Design review of the part built by this model. Coordinates are the model's own, in mm. Face numbers are marked on the shaded views. A direction names the side the tool comes from. Coordinates: 2 decimals unless noted, no trailing zeros. Write each loop counter-clockwise with the first axis right and the second up, starting at its lowest first coordinate (ties: lowest second). Pieces come first, ordered by that corner, then holes. Notation, with made-up numbers: M 59.25,52.5 L 100.25,52.5 A5 ccw 100.25,59.5 Z; hole C -19.75,39.25 d6. An arc over 180 degrees is marked long. Write item = value, one per line.
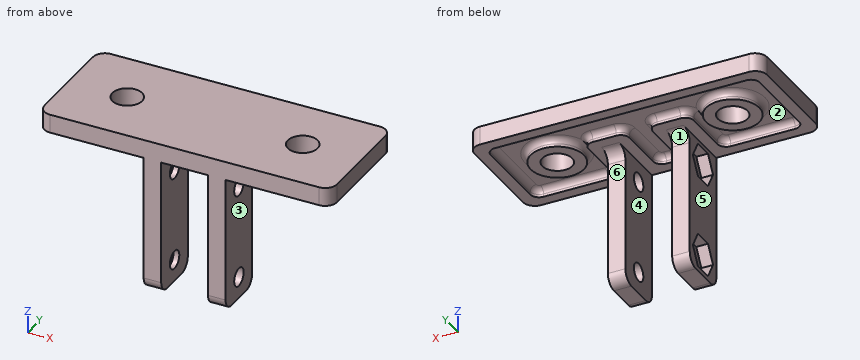
```python
from build123d import *

# Parameters (mm, degrees)
SKETCH1_W           = 50
SKETCH1_H           = 20
SKETCH1_R           = 2.55
BOSS_EXTRUDE1_DEPTH = 3.175
BOSS_EXTRUDE2_START = 4
SKETCH3_W           = 26.5
SKETCH3_H           = 8.75
SKETCH3_R           = 1.55
BOSS_EXTRUDE2_DEPTH = 3
CUT_EXTRUDE1_START  = -7
SKETCH3_3_R         = 1.55
CUT_EXTRUDE1_DEPTH  = 2
FILLET1_R           = 2
FILLET2_R           = 2
SKETCH4_R           = 4.55
CUT_EXTRUDE2_DEPTH  = 1.5
FILLET3_R           = 1.5
FILLET4_R           = 1


with BuildPart() as part:
    # Sketch1 → Boss-Extrude1 (new body)
    with BuildSketch(Plane.XY):
        Rectangle(SKETCH1_W, SKETCH1_H)
        with Locations((-15, 0)):
            Circle(SKETCH1_R, mode=Mode.SUBTRACT)
        with Locations((15, 0)):
            Circle(SKETCH1_R, mode=Mode.SUBTRACT)
    extrude(amount=BOSS_EXTRUDE1_DEPTH)

    # Sketch3 → Boss-Extrude2 (add)
    # profile 1 of 3: a face of its own
    with BuildSketch(Plane(origin=(0, 0, 0), x_dir=(0, 0, -1), z_dir=(1, 0, 0)).offset(BOSS_EXTRUDE2_START)):
        with Locations((10.075, -5.625)):
            Rectangle(SKETCH3_W, SKETCH3_H)
        Polygon((22.475, -7.259882024), (22.475, -3.940117976), (19.6, -2.280235952), (16.725, -3.940117976), (16.725, -7.259882024), (19.6, -8.919764048), align=None, mode=Mode.SUBTRACT)
        Polygon((6.475, -7.259882024), (6.475, -3.940117976), (3.6, -2.280235952), (0.725, -3.940117976), (0.725, -7.259882024), (3.6, -8.919764048), align=None, mode=Mode.SUBTRACT)
    # profile 2 of 3: a face of its own
    with BuildSketch(Plane(origin=(0, 0, 0), x_dir=(0, 0, -1), z_dir=(1, 0, 0)).offset(BOSS_EXTRUDE2_START)):
        Polygon((3.6, -8.919764048), (6.475, -7.259882024), (6.475, -3.940117976), (3.6, -2.280235952), (0.725, -3.940117976), (0.725, -7.259882024), align=None)
        with Locations((3.6, -5.6)):
            Circle(SKETCH3_R, mode=Mode.SUBTRACT)
    # profile 3 of 3: a face of its own
    with BuildSketch(Plane(origin=(0, 0, 0), x_dir=(0, 0, -1), z_dir=(1, 0, 0)).offset(BOSS_EXTRUDE2_START)):
        Polygon((19.6, -8.919764048), (22.475, -7.259882024), (22.475, -3.940117976), (19.6, -2.280235952), (16.725, -3.940117976), (16.725, -7.259882024), align=None)
        with Locations((19.6, -5.6)):
            Circle(SKETCH3_R, mode=Mode.SUBTRACT)
    boss_extrude2 = extrude(amount=BOSS_EXTRUDE2_DEPTH)

    # Mirror1: Boss-Extrude2 across plane
    add(boss_extrude2.mirror(Plane(origin=(0, 0, 0), x_dir=(0, 0, 1), z_dir=(1, 0, 0))))

    # Sketch3<3> → Cut-Extrude1 (cut)
    # profile 1 of 2: a face of its own
    with BuildSketch(Plane(origin=(0, 0, 0), x_dir=(0, 0, -1), z_dir=(1, 0, 0)).offset(CUT_EXTRUDE1_START)):
        Polygon((3.6, -8.919764048), (6.475, -7.259882024), (6.475, -3.940117976), (3.6, -2.280235952), (0.725, -3.940117976), (0.725, -7.259882024), align=None)
        with Locations((3.6, -5.6)):
            Circle(SKETCH3_3_R, mode=Mode.SUBTRACT)
    # profile 2 of 2: a face of its own
    with BuildSketch(Plane(origin=(0, 0, 0), x_dir=(0, 0, -1), z_dir=(1, 0, 0)).offset(CUT_EXTRUDE1_START)):
        Polygon((19.6, -8.919764048), (22.475, -7.259882024), (22.475, -3.940117976), (19.6, -2.280235952), (16.725, -3.940117976), (16.725, -7.259882024), align=None)
        with Locations((19.6, -5.6)):
            Circle(SKETCH3_3_R, mode=Mode.SUBTRACT)
    extrude(amount=CUT_EXTRUDE1_DEPTH, mode=Mode.SUBTRACT)

    # Fillet1
    fillet1_edges = [part.edges().sort_by_distance(p)[0] for p in [
        (5.5, -1.25, 0),
        (-5.5, -1.25, 0),
    ]]
    fillet(fillet1_edges, radius=FILLET1_R)

    # Fillet2
    fillet2_edges = [part.edges().sort_by_distance(p)[0] for p in [
        (5.5, -10, -23.325),
        (5.5, -1.25, -23.325),
        (-5.5, -10, -23.325),
        (-5.5, -1.25, -23.325),
        (25, -10, 1.5875),
        (-25, -10, 1.5875),
        (-25, 10, 1.5875),
        (25, 10, 1.5875),
    ]]
    fillet(fillet2_edges, radius=FILLET2_R)

    # Sketch4 → Cut-Extrude2 (cut)
    with BuildSketch(Plane(origin=(0, 0, 0), x_dir=(-1, 0, 0), z_dir=(0, 0, -1))):
        Polygon((9, 2.75), (9, -8), (23, -8), (23, 8), (-23, 8), (-23, -8), (-9, -8), (-9, 2.75), (-2, 2.75), (-2, -8), (2, -8), (2, 2.75), align=None)
        with Locations((15, 0)):
            Circle(SKETCH4_R, mode=Mode.SUBTRACT)
        with Locations((-15, 0)):
            Circle(SKETCH4_R, mode=Mode.SUBTRACT)
    extrude(amount=-CUT_EXTRUDE2_DEPTH, mode=Mode.SUBTRACT)

    # Fillet3
    fillet3_edges = [part.edges().sort_by_distance(p)[0] for p in [
        (-9, -8, 0.75),
        (-9, 2.75, 0.75),
        (-2, 2.75, 0.75),
        (-2, -8, 0.75),
        (2, -8, 0.75),
        (2, 2.75, 0.75),
        (9, 2.75, 0.75),
        (9, -8, 0.75),
        (23, -8, 0.75),
        (23, 8, 0.75),
        (-23, 8, 0.75),
        (-23, -8, 0.75),
    ]]
    fillet(fillet3_edges, radius=FILLET3_R)

    # Fillet4
    # the kernel refuses this fillet: 1 mm, written as the material it adds along each edge
    with BuildSketch(Plane(origin=(-15, 0, 1.5), x_dir=(-1, 0, 0), z_dir=(0, -1, 0))) as fillet4_piece_1:
        with BuildLine():
            CenterArc((4.55 + FILLET4_R, FILLET4_R), FILLET4_R, 180, 90)
            Line((4.55, FILLET4_R), (4.55, 0))
            Line((4.55, 0), (4.55 + FILLET4_R, 0))
        make_face()
    revolve(axis=Axis((-15, 0, 1.5), (0, 0, -1)))
    with BuildSketch(Plane(origin=(15, 0, 1.5), x_dir=(-1, 0, 0), z_dir=(0, -1, 0))) as fillet4_piece_2:
        with BuildLine():
            CenterArc((4.55 + FILLET4_R, FILLET4_R), FILLET4_R, 180, 90)
            Line((4.55, FILLET4_R), (4.55, 0))
            Line((4.55, 0), (4.55 + FILLET4_R, 0))
        make_face()
    revolve(axis=Axis((15, 0, 1.5), (0, 0, -1)))
    with BuildSketch(Plane(origin=(-9, 1.25, 1.5), x_dir=(0, 0, -1), z_dir=(0, -1, 0)), Plane(origin=(-2, -6.5, 1.5), x_dir=(0, 0, -1), z_dir=(0, 1, 0)), Plane(origin=(9, -6.5, 1.5), x_dir=(0, 0, -1), z_dir=(0, 1, 0)), Plane(origin=(2, 1.25, 1.5), x_dir=(0, 0, -1), z_dir=(0, -1, 0))) as fillet4_piece_3:
        with BuildLine():
            CenterArc((FILLET4_R, -FILLET4_R), FILLET4_R, 90, 90)
            Line((0, -FILLET4_R), (0, 0))
            Line((0, 0), (FILLET4_R, 0))
        make_face()
    extrude(amount=7.75)
    with BuildSketch(Plane(origin=(-3.5, 2.75, 1.5), x_dir=(0, 0, -1), z_dir=(-1, 0, 0)), Plane(origin=(7.5, 2.75, 1.5), x_dir=(0, 0, -1), z_dir=(-1, 0, 0))) as fillet4_piece_4:
        with BuildLine():
            CenterArc((FILLET4_R, -FILLET4_R), FILLET4_R, 90, 90)
            Line((0, -FILLET4_R), (0, 0))
            Line((0, 0), (FILLET4_R, 0))
        make_face()
    extrude(amount=4)
    with BuildSketch(Plane(origin=(0.5, -8, 1.5), x_dir=(0, 0, -1), z_dir=(-1, 0, 0))) as fillet4_piece_5:
        with BuildLine():
            CenterArc((FILLET4_R, -FILLET4_R), FILLET4_R, 90, 90)
            Line((0, -FILLET4_R), (0, 0))
            Line((0, 0), (FILLET4_R, 0))
        make_face()
    extrude(amount=1)
    with BuildSketch(Plane(origin=(-10.5, -8, 1.5), x_dir=(0, 0, -1), z_dir=(-1, 0, 0)), Plane(origin=(21.5, -8, 1.5), x_dir=(0, 0, -1), z_dir=(-1, 0, 0))) as fillet4_piece_6:
        with BuildLine():
            CenterArc((FILLET4_R, -FILLET4_R), FILLET4_R, 90, 90)
            Line((0, -FILLET4_R), (0, 0))
            Line((0, 0), (FILLET4_R, 0))
        make_face()
    extrude(amount=11)
    with BuildSketch(Plane(origin=(-23, -6.5, 1.5), x_dir=(0, 0, -1), z_dir=(0, 1, 0)), Plane(origin=(23, 6.5, 1.5), x_dir=(0, 0, -1), z_dir=(0, -1, 0))) as fillet4_piece_7:
        with BuildLine():
            CenterArc((FILLET4_R, -FILLET4_R), FILLET4_R, 90, 90)
            Line((0, -FILLET4_R), (0, 0))
            Line((0, 0), (FILLET4_R, 0))
        make_face()
    extrude(amount=13)
    with BuildSketch(Plane(origin=(-21.5, 8, 1.5), x_dir=(0, 0, -1), z_dir=(1, 0, 0))) as fillet4_piece_8:
        with BuildLine():
            CenterArc((FILLET4_R, -FILLET4_R), FILLET4_R, 90, 90)
            Line((0, -FILLET4_R), (0, 0))
            Line((0, 0), (FILLET4_R, 0))
        make_face()
    extrude(amount=43)
    with BuildSketch(Plane(origin=(21.5, 6.5, 1.5), x_dir=(1, 0, 0), z_dir=(0, -1, 0))) as fillet4_piece_9:
        with BuildLine():
            CenterArc((1.5 - FILLET4_R, -FILLET4_R), FILLET4_R, 0, 90)
            Line((1.5 - FILLET4_R, 0), (1.5, 0))
            Line((1.5, 0), (1.5, -FILLET4_R))
        make_face()
    revolve(axis=Axis((21.5, 6.5, 1.5), (0, 0, 1)), revolution_arc=90)
    with BuildSketch(Plane(origin=(-10.5, -6.5, 1.5), x_dir=(0, -1, 0), z_dir=(-1, 0, 0))) as fillet4_piece_10:
        with BuildLine():
            CenterArc((1.5 - FILLET4_R, -FILLET4_R), FILLET4_R, 0, 90)
            Line((1.5 - FILLET4_R, 0), (1.5, 0))
            Line((1.5, 0), (1.5, -FILLET4_R))
        make_face()
    revolve(axis=Axis((-10.5, -6.5, 1.5), (0, 0, 1)), revolution_arc=90)
    with BuildSketch(Plane(origin=(-21.5, -6.5, 1.5), x_dir=(-1, 0, 0), z_dir=(0, 1, 0))) as fillet4_piece_11:
        with BuildLine():
            CenterArc((1.5 - FILLET4_R, -FILLET4_R), FILLET4_R, 0, 90)
            Line((1.5 - FILLET4_R, 0), (1.5, 0))
            Line((1.5, 0), (1.5, -FILLET4_R))
        make_face()
    revolve(axis=Axis((-21.5, -6.5, 1.5), (0, 0, 1)), revolution_arc=90)
    with BuildSketch(Plane(origin=(-21.5, 6.5, 1.5), x_dir=(0, 1, 0), z_dir=(1, 0, 0))) as fillet4_piece_12:
        with BuildLine():
            CenterArc((1.5 - FILLET4_R, -FILLET4_R), FILLET4_R, 0, 90)
            Line((1.5 - FILLET4_R, 0), (1.5, 0))
            Line((1.5, 0), (1.5, -FILLET4_R))
        make_face()
    revolve(axis=Axis((-21.5, 6.5, 1.5), (0, 0, 1)), revolution_arc=90)
    with BuildSketch(Plane(origin=(21.5, -6.5, 1.5), x_dir=(0, -1, 0), z_dir=(-1, 0, 0))) as fillet4_piece_13:
        with BuildLine():
            CenterArc((1.5 - FILLET4_R, -FILLET4_R), FILLET4_R, 0, 90)
            Line((1.5 - FILLET4_R, 0), (1.5, 0))
            Line((1.5, 0), (1.5, -FILLET4_R))
        make_face()
    revolve(axis=Axis((21.5, -6.5, 1.5), (0, 0, 1)), revolution_arc=90)
    with BuildSketch(Plane(origin=(10.5, -6.5, 1.5), x_dir=(-1, 0, 0), z_dir=(0, 1, 0))) as fillet4_piece_14:
        with BuildLine():
            CenterArc((1.5 - FILLET4_R, -FILLET4_R), FILLET4_R, 0, 90)
            Line((1.5 - FILLET4_R, 0), (1.5, 0))
            Line((1.5, 0), (1.5, -FILLET4_R))
        make_face()
    revolve(axis=Axis((10.5, -6.5, 1.5), (0, 0, 1)), revolution_arc=90)
    with BuildSketch(Plane(origin=(0.5, -6.5, 1.5), x_dir=(0, -1, 0), z_dir=(-1, 0, 0))) as fillet4_piece_15:
        with BuildLine():
            CenterArc((1.5 - FILLET4_R, -FILLET4_R), FILLET4_R, 0, 90)
            Line((1.5 - FILLET4_R, 0), (1.5, 0))
            Line((1.5, 0), (1.5, -FILLET4_R))
        make_face()
    revolve(axis=Axis((0.5, -6.5, 1.5), (0, 0, 1)), revolution_arc=90)
    with BuildSketch(Plane(origin=(-0.5, -6.5, 1.5), x_dir=(-1, 0, 0), z_dir=(0, 1, 0))) as fillet4_piece_16:
        with BuildLine():
            CenterArc((1.5 - FILLET4_R, -FILLET4_R), FILLET4_R, 0, 90)
            Line((1.5 - FILLET4_R, 0), (1.5, 0))
            Line((1.5, 0), (1.5, -FILLET4_R))
        make_face()
    revolve(axis=Axis((-0.5, -6.5, 1.5), (0, 0, 1)), revolution_arc=90)
    with BuildSketch(Plane(origin=(-7.5, 1.25, 1.5), x_dir=(0, 1, 0), z_dir=(1, 0, 0))) as fillet4_piece_17:
        with BuildLine():
            CenterArc((1.5 + FILLET4_R, -FILLET4_R), FILLET4_R, 90, 90)
            Line((1.5 + FILLET4_R, 0), (1.5, 0))
            Line((1.5, 0), (1.5, -FILLET4_R))
        make_face()
    revolve(axis=Axis((-7.5, 1.25, 1.5), (0, 0, 1)), revolution_arc=90)
    with BuildSketch(Plane(origin=(-3.5, 1.25, 1.5), x_dir=(0, 1, 0), z_dir=(-1, 0, 0))) as fillet4_piece_18:
        with BuildLine():
            CenterArc((1.5 + FILLET4_R, FILLET4_R), FILLET4_R, 180, 90)
            Line((1.5 + FILLET4_R, 0), (1.5, 0))
            Line((1.5, 0), (1.5, FILLET4_R))
        make_face()
    revolve(axis=Axis((-3.5, 1.25, 1.5), (0, 0, -1)), revolution_arc=90)
    with BuildSketch(Plane(origin=(3.5, 1.25, 1.5), x_dir=(-1, 0, 0), z_dir=(0, -1, 0))) as fillet4_piece_19:
        with BuildLine():
            CenterArc((1.5 + FILLET4_R, FILLET4_R), FILLET4_R, 180, 90)
            Line((1.5 + FILLET4_R, 0), (1.5, 0))
            Line((1.5, 0), (1.5, FILLET4_R))
        make_face()
    revolve(axis=Axis((3.5, 1.25, 1.5), (0, 0, -1)), revolution_arc=90)
    with BuildSketch(Plane(origin=(7.5, 1.25, 1.5), x_dir=(0, 1, 0), z_dir=(-1, 0, 0))) as fillet4_piece_20:
        with BuildLine():
            CenterArc((1.5 + FILLET4_R, FILLET4_R), FILLET4_R, 180, 90)
            Line((1.5 + FILLET4_R, 0), (1.5, 0))
            Line((1.5, 0), (1.5, FILLET4_R))
        make_face()
    revolve(axis=Axis((7.5, 1.25, 1.5), (0, 0, -1)), revolution_arc=90)


solid = part.part
```
Q1. Consider section B-B, the plane z = -20.5. State the section outline as (x, y) points, and give its area (3 significant figures).
Check result:
outline = M -7,-10 L -4,-10 L -4,-6.86 L -5,-6.86 L -5,-8.4 L -7,-8.4 Z; M -7,-2.8 L -5,-2.8 L -5,-4.34 L -4,-4.34 L -4,-1.25 L -7,-1.25 Z; M 4,-10 L 7,-10 L 7,-6.86 L 4,-6.86 Z; M 4,-4.34 L 7,-4.34 L 7,-1.25 L 4,-1.25 Z
area = 31.2 mm²
Q2. The part is to be moulded in two halves that separate along X. For the marked faces 1, 2 and 3, say which applies: +X half, -X half, draft (parallel to the pull), parting line (faces both ways), or undercut.
Check result:
face_1 = draft
face_2 = undercut
face_3 = +X half
Q3. For P1, Ø6.5, axis at y = -5, z = -20.5, coming from the -X side; P2, Ø4, axis at y = -5.6, z = -3.6, coming from the -X side; P3, Ø1.5, axis at x = -5, z = -13.5, coming from the +Y side; P4, Ø1, axis at y = -0.5, z = -10, coming from the -X side (3 decimals), all flat-tipped, find the tip position at first contact; note any pin that passes through.
Check result:
P1 = -7
P2 = -5
P3 = -1.25
P4 = through
Q4. Machinability: for the marked faces 4, 5 and 6, which of the approach directions +Z, -Z, +X, -X, +Y, -Y give a long, thin tool a straight path to every point of the face, cutting with its end or side? Answer none if there is none.
Check result:
face_4 = -Z, +Y, -Y
face_5 = -Z, -X, +Y, -Y
face_6 = -Z, +X, -X, +Y
Q5. Wall thickness on line 1 (X direction, y = -2.75, z = -19.25); line 2 (X direction, y = -7, z = -9); line 3 (X direction, y = -6, z = 1.25): over which ranges is each line inside the solid? List them lowest first.
Check result:
line_1 = -5 to -4, 4 to 7
line_2 = -7 to -4, 4 to 7
line_3 = -25 to -22.66, -9.34 to -1.66, 1.66 to 9.34, 22.66 to 25
Q6. Consider section A-A, the plane z = -15.75. State the section outline as (x, y) points, and give its area (3 significant figures).
Check result:
outline = M -7,-10 L -4,-10 L -4,-1.25 L -7,-1.25 Z; M 4,-10 L 7,-10 L 7,-1.25 L 4,-1.25 Z
area = 52.5 mm²
Q7. Consider section C-C, the plane y = 0. State how many separate pieces and enclosed holes the cut face has, and give its area (3 significant figures).
Check result:
separate_pieces = 3
enclosed_holes = 0
area = 109 mm²
